Input: part model. Units: mm. Frame: model coordinates. A direction names the side the tool comes from. Give positions to 0.01 mm unless a question says otherwise; leave off trailing zeros. Write each loop counter-clockwise with the first axis right and the second up, starting at its lowest first coordinate (ties: lowest second). Pieces come first, ordered by that corner, then holes. Notation, with made-up numbers: (50.25, 13.5) - (89.25, 13.5) arc R22 cw to (89.25, 31.5) - close; hole circle Ø6 at (50, 71.25). An arc over 180 degrees is marked (long way). Answer as CSV lines item,"result".
```python
from build123d import *

# Parameters (mm, degrees)
F0_R     = 6.35
F1_DEPTH = 16.002
F2_DEPTH = 45.974
F4_DEPTH = 25.4
F5_DEPTH = 25.4


with BuildPart() as f1:
    # F0 (on Front) → F1 (new body)
    with BuildSketch(Plane.XZ):
        with BuildLine():
            ThreePointArc((76.2, 28.448), (74.593204, 13.873955), (69.85, 0))
            Line((69.85, 0), (101.6, 0))
            Line((101.6, 0), (101.6, 28.448))
            ThreePointArc((101.6, 28.448), (88.9, 41.148), (76.2, 28.448))
        make_face()
        with Locations((88.9, 28.448)):
            Circle(F0_R, mode=Mode.SUBTRACT)
        with BuildLine():
            Line((0, 28.448), (0, 0))
            Line((0, 0), (31.75, 0))
            ThreePointArc((31.75, 0), (27.006796, 13.873955), (25.4, 28.448))
            ThreePointArc((25.4, 28.448), (12.7, 41.148), (0, 28.448))
        make_face()
        with Locations((12.7, 28.448)):
            Circle(F0_R, mode=Mode.SUBTRACT)
    extrude(amount=F1_DEPTH)

    # F0 (on Front) → F2 (join)
    with BuildSketch(Plane.XZ):
        Polygon((31.75, 0), (0, 0), (0, -16.002), (101.6, -16.002), (101.6, 0), (69.85, 0), align=None)
    extrude(amount=F2_DEPTH)

    # F3 (on face) → F4 (cut)
    with BuildSketch(Plane.XY):
        with BuildLine():
            ThreePointArc((31.75, -45.974), (21.985897, -42.09333), (17.549587, -32.56881))
            ThreePointArc((17.549587, -32.56881), (12.066972, -20.797928), (0, -16.002))
            Line((0, -16.002), (0, -45.974))
            Line((0, -45.974), (31.75, -45.974))
        make_face()
        with BuildLine():
            ThreePointArc((84.050413, -32.56881), (79.614103, -42.09333), (69.85, -45.974))
            Line((69.85, -45.974), (101.6, -45.974))
            Line((101.6, -45.974), (101.6, -16.002))
            ThreePointArc((101.6, -16.002), (89.533028, -20.797928), (84.050413, -32.56881))
        make_face()
    extrude(amount=-F4_DEPTH, mode=Mode.SUBTRACT)

    # F3 (on face) → F5 (cut)
    with BuildSketch(Plane.XY):
        with BuildLine():
            Line((31.75, -38.1), (69.85, -38.1))
            ThreePointArc((69.85, -38.1), (76.2, -31.75), (69.85, -25.4))
            Line((69.85, -25.4), (31.75, -25.4))
            ThreePointArc((31.75, -25.4), (25.4, -31.75), (31.75, -38.1))
        make_face()
    extrude(amount=-F5_DEPTH, mode=Mode.SUBTRACT)


solid = f1.part
```
Item 1: Cut plane B-B on y = -6. Return the cut outline in (x, z), plus the area to 3 significant figures.
The answers:
outline,"(0, -16) - (101.6, -16) - (101.6, 28.45) arc R12.7 ccw to (76.2, 28.45) arc R66.9 cw to (69.85, 0) - (31.75, 0) arc R66.9 cw to (25.4, 28.45) arc R12.7 ccw to (0, 28.45) - close; hole circle Ø12.7 at (12.7, 28.45); hole circle Ø12.7 at (88.9, 28.45)"
area,"3,440 mm²"
Item 2: Mould query, pull axis X, two halves, no side actions, for faces 1 (the face through (50, -18, -16.002)), 2 (the face through (89.67, -20.67, -7.89)), 3 (the face through (74.638, -7.889, 14.075)). Classes: +X half, -X half, draft (parallel to the pull), parting line (faces both ways), or undercut.
The answers:
face 1,"draft"
face 2,"+X half"
face 3,"undercut"
Item 3: Cut plane A-A on x = 36.5. Return the cut outline in (y, z).
The answers:
outline,"(-45.97, -16) - (-38.1, -16) - (-38.1, 0) - (-45.97, 0) - close; (-25.4, -16) - (0, -16) - (0, 0) - (-25.4, 0) - close"
Item 4: Cut plane D-D on z = -3.5. Return the cut outline in (x, y).
The answers:
outline,"(0, -16) arc R17.58 cw to (17.55, -32.57) arc R14.22 ccw to (31.75, -45.97) - (69.85, -45.97) arc R14.22 ccw to (84.05, -32.57) arc R17.58 cw to (101.6, -16) - (101.6, 0) - (0, 0) - close; hole (31.75, -38.1) - (69.85, -38.1) arc R6.35 ccw to (69.85, -25.4) - (31.75, -25.4) arc R6.35 ccw to start"
Item 5: Contact query for flat-ended pins moving along their axis: pin 1 (5 mm diameter, centred on y = -36, z = -8.5, fed in from -X); pin 2 (5 mm diameter, centred on x = 58, z = -5.5, fed in from +Y); pin 3 (1.5 mm diameter, centred on x = 22.5, z = 16, fed in from -Y); pin 4 (2 mm diameter, centred on x = 47, y = -13.5, fed in from +Z). Output: stop coordinate, or through.
The answers:
pin 1,"x = 17.63"
pin 2,"y = 0"
pin 3,"y = -16"
pin 4,"z = 0"
Item 6: Reachability of faces 4 (the face through (89, -16.002, 16)), 5 (the face through (27.052, -7.889, 13.673)), 6 (the face through (50, 0, -6)), 7 (the face through (76.2, -31.9, -7.9)) from +Z, -Z, +X, -X, +Y, -Y: full face, straight path, thin tool, end or side. Return the list, or none.
The answers:
face 4,"+Z, +X, -X, -Y"
face 5,"+Z, +Y, -Y"
face 6,"+Z, -Z, +X, -X, +Y"
face 7,"+Z, -Z"
Item 7: Ray query, line 1 (Z direction, x = 88.9, y = -5.75); line 2 (X direction, y = -7.5, z = 31); line 3 (Z direction, x = 66, y = -12). Return the intervals inside material, ascending. Write a range as from..to.
The answers:
line 1,"-16..22.1, 34.8..41.15"
line 2,"0.26..6.89, 18.51..25.14, 76.46..83.09, 94.71..101.34"
line 3,"-16..0"
Item 8: Cut plane C-C on z = 13. Return the cut outline in (x, y).
The answers:
outline,"(0, -16) - (27.21, -16) - (27.21, 0) - (0, 0) - close; (74.39, -16) - (101.6, -16) - (101.6, 0) - (74.39, 0) - close"
